Source: CAD feature listing. Evaluate the final solid. Frame: model axes, mm. A direction names the side the tool comes from. Round coordinates to 2 decimals unless told otherwise and drop trailing zeros. Order: outer loops, then holes, each group sorted by start corner. A loop starts at its lowest first (then second) coordinate and runs counter-clockwise, first axis right, second up. Notation, with made-up numbers: (-20.5, 83.25) - (12.5, 83.25) arc R21 cw to (12.5, 110.25) - close; hole circle Ø10 at (44, -36). An arc over 180 degrees is marked (long way). Return JSON: item names as keys, results as strings. Group by question number.
1) Access query for faces 5 (the flat face through (0, 0.5, -0.7)), 6 (the flat face through (-2, 1.5, -2)), 7 (the flat face through (0, 0.5, -8.6)), 8 (the flat face through (1, 0.7, -4.4)). Directions: +Z, -Z, +X, -X, +Y, -Y. A direction counts if a zero-diameter tool reaches every point of the face in a straight line with its end or side. Return the directions, or none.
2) Contact query for flat-ended pins moving along their axis: P1, Ø0.7, axis at y = 1.5, z = -6.5, coming from the -X side; P2, Ø2, axis at x = -9.5, z = -7, coming from the +Y side; P3, Ø1.1, axis at y = 0.5, z = -0.5, coming from the +X side; P4, Ø1.1, axis at x = -0.5, y = 1, coming from the +Z side. Output: stop coordinate, or through.
3) Ray query, line 1 (Y direction, x = -14.25, z = -6.25); line 2 (X direction, y = 1.1, z = -2); line 3 (X direction, y = 0.6, z = -0.75). Return the intervals inside material, ascending. Write a range as from..to.
4) Section A-A, the plane y = 1.9. Return loops of the section in (x, z).
5) Section B-B, the plane x = -8. Return loops of the section in (y, z), plus the area to 3 significant figures.
6) Mould query, pull axis Z, two halves, no side actions, for faces 1 (the cylindrical face through (-5.64, 0.96, -4.15)), 2 (the flat face through (-12.6, 0.5, -9.8)), 3 (the flat face through (-2, 1.5, -6.7)), 4 (the flat face through (-12.6, 0.5, 0)). Classes: pulls with the +Z half, pulls with the -Z half, needs draft (parallel to the pull), parting line crosses it, or undercut.
7) Section C-C, the plane z = -3. Return loops of the section in (x, y), plus the area to 3 significant figures.
```python
from build123d import *

# Parameters (mm, degrees)
SKETCH1_W           = 24.8
SKETCH1_H           = 9.8
BOSS_EXTRUDE1_DEPTH = 1
SKETCH2_W           = 3
SKETCH2_H           = 6.1
BOSS_EXTRUDE2_DEPTH = 3.25
SKETCH4_W           = 1
SKETCH4_H           = 6.1
BOSS_EXTRUDE3_DEPTH = 1
SKETCH3_R           = 3.3
CUT_EXTRUDE1_DEPTH  = 21.25
FILLET1_R           = 0.2


with BuildPart() as part:
    # Sketch1 → Boss-Extrude1 (new body)
    with BuildSketch(Plane(origin=(0, 0, 0), x_dir=(1, 0, 0), z_dir=(0, 1, 0))):
        with Locations((-12.4, 4.9)):
            Rectangle(SKETCH1_W, SKETCH1_H)
    extrude(amount=BOSS_EXTRUDE1_DEPTH)

    # Sketch2 → Boss-Extrude2 (add)
    with BuildSketch(Plane(origin=(0, 1, 0), x_dir=(1, 0, 0), z_dir=(0, 1, 0))):
        with Locations((-0.5, 4.4)):
            Rectangle(SKETCH2_W, SKETCH2_H)
    extrude(amount=BOSS_EXTRUDE2_DEPTH)

    # Sketch4 → Boss-Extrude3 (add)
    with BuildSketch(Plane.XZ.offset(-1)):
        with Locations((0.5, -4.4)):
            Rectangle(SKETCH4_W, SKETCH4_H)
    extrude(amount=BOSS_EXTRUDE3_DEPTH)

    # Sketch3 → Cut-Extrude1 (cut)
    with BuildSketch(Plane(origin=(1, 0, 0), x_dir=(0, 0, -1), z_dir=(1, 0, 0))):
        with Locations((4.4, 4.25)):
            Circle(SKETCH3_R)
    extrude(amount=-CUT_EXTRUDE1_DEPTH, mode=Mode.SUBTRACT)

    # Fillet1
    fillet1_edges = [part.edges().sort_by_distance(p)[0] for p in [
        (-0.5, 2.990039683, -1.35),
        (-0.5, 2.990039683, -7.45),
    ]]
    fillet(fillet1_edges, radius=FILLET1_R)


solid = part.part
```
Geometry check:
{
 "1": {"face 5": "+Z, +X, +Y, -Y", "face 6": "+Z, -Z, -X, +Y", "face 7": "-Z, +X, +Y, -Y", "face 8": "+Z, -Z, +X, +Y, -Y"},
 "2": {"P1": "x = -2", "P2": "y = 1", "P3": "x = 0", "P4": "z = 0"},
 "3": {"line 1": "0..1", "line 2": "-2..1", "line 3": "-24.8..0"},
 "4": {"outline": "(-2, -7.45) - (1, -7.45) - (1, -6.72) - (-2, -6.72) - close; (-2, -2.08) - (1, -2.08) - (1, -1.35) - (-2, -1.35) - close"},
 "5": {"outline": "(0, -9.8) - (1, -9.8) - (1, -4.97) arc R3.3 cw to (1, -3.83) - (1, 0) - (0, 0) - close", "area": "9.76 mm2"},
 "6": {"face 1": "undercut", "face 2": "pulls with the -Z half", "face 3": "needs draft", "face 4": "pulls with the +Z half"},
 "7": {"outline": "(-24.8, 0) - (1, 0) - (1, 1.26) - (-2, 1.26) - (-2, 1) - (-24.8, 1) - close", "area": "26.6 mm2"}
}
